Design review of the part built by this model. Coordinates are the model's own, in mm. Face numbers are marked on the shaded views. A direction names the side the tool comes from. Give positions to 0.01 mm unless a question says otherwise; leave off trailing zeros. Write each loop counter-clockwise with the first axis right and the second up, starting at its lowest first coordinate (ties: lowest second). Pieces come first, ordered by that corner, then holes.
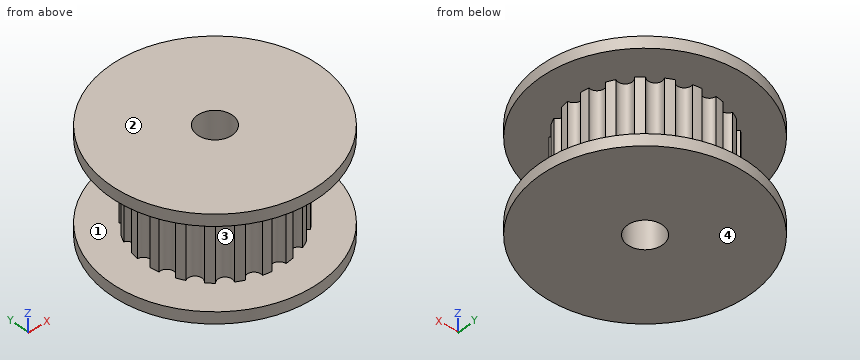
```python
from build123d import *

# Parameters (mm, degrees)
SKETCH_1_R               = 9
EXTRUDE_1_DEPTH          = 0.5
SKETCH_2_R               = 6.115
EXTRUDE_2_DEPTH          = 7
CUT_EXTRUDE_3_DEPTH      = 7
SKETCH_3_R               = 9
EXTRUDE_3_DEPTH          = 1
SKETCH_6_R               = 1.5
CUT_EXTRUDE_2_DEPTH      = 10
PATTERN_CIRCULAR_2_COUNT = 20


with BuildPart() as part:
    # 草圖1 → 填料-伸長1 (new body, symmetric)
    with BuildSketch(Plane.XY):
        Circle(SKETCH_1_R)
    extrude(amount=EXTRUDE_1_DEPTH, both=True)

    # 草圖2 → 填料-伸長2 (add)
    with BuildSketch(Plane.XY.offset(0.5)):
        Circle(SKETCH_2_R)
    extrude(amount=EXTRUDE_2_DEPTH)

    # 草圖7 → 除料-伸長3 (cut)
    with BuildSketch(Plane.XY.offset(7.5)):
        with BuildLine():
            ThreePointArc((-0.599277509, 6.085564186), (0, 5.515), (0.599277509, 6.085564186))
            ThreePointArc((0.599277509, 6.085564186), (0, 6.115), (-0.599277509, 6.085564186))
        make_face()
    cut_extrude_3 = extrude(amount=-CUT_EXTRUDE_3_DEPTH, mode=Mode.SUBTRACT)

    # 草圖3 → 填料-伸長3 (add)
    with BuildSketch(Plane.XY.offset(7.5)):
        Circle(SKETCH_3_R)
    extrude(amount=EXTRUDE_3_DEPTH)

    # 草圖6 → 除料-伸長2 (cut, through all)
    with BuildSketch(Plane(origin=(0, 0, -0.5), x_dir=(-1, 0, 0), z_dir=(0, 0, -1))):
        Circle(SKETCH_6_R)
    extrude(amount=-CUT_EXTRUDE_2_DEPTH, mode=Mode.SUBTRACT)

    # 環狀複製排列2: 除料-伸長3 ×20 about axis
    pattern_circular_2_axis = Axis((0, 0, 0), (0, 0, 1))
    for i in range(1, PATTERN_CIRCULAR_2_COUNT):
        add(cut_extrude_3.rotate(pattern_circular_2_axis, i * 360 / PATTERN_CIRCULAR_2_COUNT), mode=Mode.SUBTRACT)


solid = part.part
```
(1) To check wall thickness, follow L1, parallel to Z at x = -5, y = 7.25; L2, parallel to Y at x = 0, z = 6.75 (3 decimals); L3, parallel to Y at x = -0.75, z = 5.5. State the ranges of each line that lie inside material, in increasing order.
Resolved:
L1: z = -0.5 to 0.5, 7.5 to 8.5
L2: y = -5.515 to -1.5, 1.5 to 5.515
L3: y = -6.07 to -1.3, 1.3 to 6.07
(2) Clearance check with flat-ended pins moving along their axes: P1, Ø2, axis at y = 2, z = 2, coming from the +X side; P2, Ø4, axis at y = 2, z = 4, coming from the +X side; P3, Ø1.5, axis at y = 3.5, z = 3, coming from the +X side; P4, Ø3.5, axis at x = 0, y = 0, coming from the +Z side. State where each tip first meets the part, or that it passes through.
Resolved:
P1: stops at x = 6.03
P2: stops at x = 6.09
P3: stops at x = 5.46
P4: stops at z = 8.5
(3) Tool access review of the marked faces 1 and 2: name each direction out of +Z, -Z, +X, -X, +Y, -Y from which nothing blocks a thin tool from reaching the whole face with its end or side.
Resolved:
face 1: none
face 2: +Z, +X, -X, +Y, -Y
(4) Mouldability with a two-part tool opening along X and no side actions: class the marked faces 3 and 4 as pulls with the +X half, pulls with the -X half, needs draft (parallel to the pull), parting line crosses it, or undercut.
Resolved:
face 3: undercut
face 4: needs draft
(5) Consider section A-A, the plane y = 0. Give the boundary of the cut face in (x, z) (3 decimals), then the cut area to 3 significant figures.
Resolved:
outline: (-9, -0.5) - (-1.5, -0.5) - (-1.5, 8.5) - (-9, 8.5) - (-9, 7.5) - (-5.515, 7.5) - (-5.515, 0.5) - (-9, 0.5) - close; (1.5, -0.5) - (9, -0.5) - (9, 0.5) - (5.515, 0.5) - (5.515, 7.5) - (9, 7.5) - (9, 8.5) - (1.5, 8.5) - close
area: 86.2 mm2
(6) Consider section C-C, the plane z = 8.25. Give the boundary of the cut face in (x, y).
Resolved:
outline: circle Ø18 at (0, 0); hole circle Ø3 at (0, 0)
(7) Consider section D-D, the plane x = -3.75. Give the boundary of the cut face in (y, z).
Resolved:
outline: (-8.18, -0.5) - (8.18, -0.5) - (8.18, 0.5) - (4.37, 0.5) - (4.37, 7.5) - (8.18, 7.5) - (8.18, 8.5) - (-8.18, 8.5) - (-8.18, 7.5) - (-4.37, 7.5) - (-4.37, 0.5) - (-8.18, 0.5) - close
